from build123d import *

# Parameters (mm, degrees)
F0_R     = 2
F1_DEPTH = 2
F3_DEPTH = 24
F4_R     = 2
F5_DEPTH = 4
F6_DEPTH = 4
F8_DEPTH = 10


with BuildPart() as f1:
    # F0 (on Top) → F1 (new body)
    with BuildSketch(Plane.XY):
        with BuildLine():
            Line((8, 0), (0, 0))
            Line((0, 0), (0, -8))
            ThreePointArc((0, -8), (4, -12), (8, -8))
            Line((8, -8), (8, 0))
        make_face()
        with Locations((4, -8)):
            Circle(F0_R, mode=Mode.SUBTRACT)
        with BuildLine():
            Line((0, 20), (0, 0))
            Line((0, 0), (8, 0))
            Line((8, 0), (40, 0))
            ThreePointArc((40, 0), (42.8284271247, 1.1715728753), (44, 4))
            Line((44, 4), (44, 20))
            ThreePointArc((44, 20), (42.8284271247, 22.8284271247), (40, 24))
            Line((40, 24), (4, 24))
            ThreePointArc((4, 24), (1.1715728753, 22.8284271247), (0, 20))
        make_face()
        with Locations((40, 4)):
            Circle(F0_R, mode=Mode.SUBTRACT)
        with Locations((4, 20)):
            Circle(F0_R, mode=Mode.SUBTRACT)
        with Locations((40, 20)):
            Circle(F0_R, mode=Mode.SUBTRACT)
    extrude(amount=F1_DEPTH)

    # F2 (on face) → F3 (join)
    with BuildSketch(Plane.YZ.offset(8)):
        Polygon((0, 12), (0, 2), (8, 2), (8, 14.7138329376), (24.2451953819, 32.1346721534), (38.5059458821, 32.1346721534), (38.5059458821, 36.1346721534), (22.5059458821, 36.1346721534), align=None)
    extrude(amount=F3_DEPTH)

    # F4 (on face) → F5 (join)
    with BuildSketch(Plane(origin=(0, -5.9853843016, 5.5814611575), x_dir=(1, 0, 0), z_dir=(0, -0.7313537016, 0.6819983601))):
        with BuildLine():
            Line((8, 18.7762444194), (8, 30.7762444194))
            Line((8, 30.7762444194), (4, 30.7762444194))
            ThreePointArc((4, 30.7762444194), (-2, 24.7762444194), (4, 18.7762444194))
            Line((4, 18.7762444194), (8, 18.7762444194))
        make_face()
        with Locations((4, 24.7762444194)):
            Circle(F4_R, mode=Mode.SUBTRACT)
    extrude(amount=-F5_DEPTH)

    # F4 (on face) → F6 (cut, through all)
    with BuildSketch(Plane(origin=(0, -5.9853843016, 5.5814611575), x_dir=(1, 0, 0), z_dir=(0, -0.7313537016, 0.6819983601))):
        with BuildLine():
            ThreePointArc((26, 32.7762444194), (24, 34.7762444194), (22, 32.7762444194))
            Line((22, 32.7762444194), (22, 18.7762444194))
            ThreePointArc((22, 18.7762444194), (24, 16.7762444194), (26, 18.7762444194))
            Line((26, 18.7762444194), (26, 32.7762444194))
        make_face()
    extrude(amount=-F6_DEPTH, mode=Mode.SUBTRACT)

    # F7 (on face) → F8 (cut)
    with BuildSketch(Plane.XY.offset(36.1346721534)):
        with BuildLine():
            Line((14, 38.5059458821), (26, 38.5059458821))
            ThreePointArc((26, 38.5059458821), (20, 44.5059458821), (14, 38.5059458821))
        make_face()
        with BuildLine():
            ThreePointArc((14, 38.5059458821), (20, 32.5059458821), (26, 38.5059458821))
            Line((26, 38.5059458821), (14, 38.5059458821))
        make_face()
    extrude(amount=-F8_DEPTH, mode=Mode.SUBTRACT)


solid = f1.part
Part model, mm, in its own coordinate system. A direction names the side the tool comes from. Coordinates: 2 decimals unless noted, no trailing zeros. Loops run counter-clockwise (first coordinate to the right, second up) from the corner with the lowest first, then second, coordinate; pieces in that order, holes last. Notation, with made-up numbers: (52, 73) -> (64, 73) arc R34 ccw to (64, 108) -> close; hole circle Ø9 at (-12, 30). An arc over 180 degrees is marked (long way). Use a Markdown table: item, result. Add a question column.
Item 1: Band-saw the part on B-B on x = 20. Write the cut outline in (y, z), plus the area to 3 significant figures.
Item 2: Band-saw the part on D-D on y = -2. Write the cut outline in (x, z).
Item 3: Flat gauge pins, fed straight in: P1, Ø3.5, axis at x = 4, y = -8, coming from the +Z side; P2, Ø4.5, axis at x = 40, y = 4, coming from the -Z side; P3, Ø9.5, axis at x = 23.5, z = 6.5, coming from the -Y side; P4, Ø3.5, axis at y = 15.5, z = 24, coming from the -X side. Where does each tip first touch, or does it go through?
Item 4: Probe probe 1 along Y at (x, z) = (40, 1.45); probe 2 along Y at (x, z) = (4, 1.3); probe 3 along X at (y, z) = (14, 22). List the from-to ranges inside material, lowest first.
Item 5: Pull direction Z, two halves, no side cores. Call faces 1 (the flat face through (20, 30, 32.135)), 2 (the flat face through (22, 10, 2)), 3 (the cylindrical face through (-2, 12.4, 22.5)), 4 (the flat face through (8, -4, 1)): +Z half, -Z half, draft (parallel to the pull), parting line (faces both ways), or undercut.
Item 6: Band-saw the part on A-A on y = 35. Write the cut outline in (x, z), plus the area to 3 significant figures.
Item 7: Band-saw the part on C-C on z = 5. Write the cut outline in (x, y), plus the area to 3 significant figures.
Item 8: Which spindle directions (+Z, -Z, +X, -X, +Y, -Y) get a long thin tool onto all of the face, cutting with end or side? Do faces 5 (the flat face through (20, 0, 6)), 6 (the flat face through (20, 8, 8)), 7 (the flat face through (32, 13, 22)). Say none if no direction does.
Geometry says:
| question | item | result |
|---|---|---|
| 1 | outline | (0, 0) -> (24, 0) -> (24, 2) -> (8, 2) -> (8, 14.71) -> (24.25, 32.13) -> (32.51, 32.13) -> (32.51, 36.13) -> (22.51, 36.13) -> (0, 12) -> close |
| 1 | area | 289 mm² |
| 2 | outline | (0, 0) -> (8, 0) -> (8, 2) -> (0, 2) -> close |
| 3 | P1 | through |
| 3 | P2 | z = 0 |
| 3 | P3 | y = 0 |
| 3 | P4 | x = -1.78 |
| 4 | probe 1 | 0 to 2, 6 to 18, 22 to 24 |
| 4 | probe 2 | -12 to -10, -6 to 18, 22 to 24 |
| 4 | probe 3 | -1.94 to 2.2, 5.8 to 22, 26 to 32 |
| 5 | face 1 | -Z half |
| 5 | face 2 | undercut |
| 5 | face 3 | undercut |
| 5 | face 4 | draft |
| 6 | outline | (8, 32.13) -> (15.13, 32.13) -> (15.13, 36.13) -> (8, 36.13) -> close; (24.87, 32.13) -> (32, 32.13) -> (32, 36.13) -> (24.87, 36.13) -> close |
| 6 | area | 57.0 mm² |
| 7 | outline | (8, 0) -> (32, 0) -> (32, 8) -> (8, 8) -> close |
| 7 | area | 192 mm² |
| 8 | face 5 | +Z, -Z, +X, -Y |
| 8 | face 6 | +X, -X, +Y |
| 8 | face 7 | +Z, +X, +Y, -Y |
